Read the model definition and answer for the solid it produces. Units are mm, in the model's axes. A direction names the side the tool comes from. Coordinates: 2 decimals unless noted, no trailing zeros. Loops run counter-clockwise (first coordinate to the right, second up) from the corner with the lowest first, then second, coordinate; pieces in that order, holes last. Notation, with made-up numbers: (47.25, -18.5) - (76.25, -18.5) arc R6 ccw to (76.25, -9.5) - close; hole circle Ø3 at (33.5, -20.75). An arc over 180 degrees is marked (long way). Use one line per item in the form item = value.
from build123d import *

# Parameters (mm, degrees)
F1_DEPTH    = 3.81
F3_T2_ANGLE = 45.4323000541
F2_W        = 20.7137
F2_H        = 2.54
F4_DEPTH    = 30.226
F8_DEPTH    = 20.7137
F9_W        = 10.5537
F9_H        = 7.0042966513
F10_DEPTH   = 51.8170001
F6_W        = 3.81
F6_H        = 40.64
F11_DEPTH   = 10.16


# Not quite as in the source:
# - a fillet or chamfer that OpenCascade refuses, or shapes differently, is made with other operations: its cross-section is extruded or revolved along the edge and cut away or added


with BuildPart() as f1:
    # F0 (on Top) → F1 (new body)
    with BuildSketch(Plane.XY):
        with BuildLine():
            ThreePointArc((32.3535154368, 26.1046796118), (-0.7575616132, 26.3503201986), (-32.5620487044, 17.1373747646))
            Line((-32.5620487044, 17.1373747646), (32.3535154368, 26.1046796118))
        make_face()
        Polygon((32.3535154368, 26.1046796118), (-32.5620487044, 17.1373747646), (-14.3325939581, -32.94764052), (-14.3325939581, -93.2497044648), (21.0546860419, -93.2497044648), align=None)
    extrude(amount=F1_DEPTH)

    # F3: fillet of radius 5.08 on 1 edges, made by hand

    # F3_s1 → F3_t2 (revolve, cut)
    with BuildSketch(Plane(origin=(35.6245782938, -9.4464852648, 0), x_dir=(0, 0, 1), z_dir=(0.966594728, -0.2563096405, 0))):
        with BuildLine():
            ThreePointArc((3.81, -34.1830353327), (1.0639073716, -32.3751984564), (0, -29.2643464831))
            Line((0, -29.2643464831), (0, -34.1830353327))
            Line((0, -34.1830353327), (3.81, -34.1830353327))
        make_face()
    revolve(axis=Axis((14.9550445097, -87.395415893, 0), (0, 0, 1)), revolution_arc=F3_T2_ANGLE, mode=Mode.SUBTRACT)

    # F2 (on face) → F4 (join)
    with BuildSketch(Plane.XY.offset(3.81)):
        with Locations((-0.8633345632, 20.0644456113)):
            Rectangle(F2_W, F2_H)
        with Locations((-0.8633345632, -23.1155543887)):
            Rectangle(F2_W, F2_H)
    extrude(amount=F4_DEPTH)

    # F7 (on face) → F8 (join)
    with BuildSketch(Plane.YZ.offset(9.4935154368)):
        Polygon((-24.3855543887, 40.8603511751), (-24.3855543887, 34.036), (-21.8455543887, 34.036), (-20.6579078442, 34.036), align=None)
        Polygon((17.6067990667, 34.036), (21.3344456113, 34.036), (21.3344456113, 40.8603511751), align=None)
    extrude(amount=-F8_DEPTH)

    # F9 (on face) → F10 (cut, through all)
    with BuildSketch(Plane.XZ.offset(24.3855543887)):
        with Locations((-0.8633345632, 37.3582028494)):
            Rectangle(F9_W, F9_H)
    extrude(amount=-F10_DEPTH, mode=Mode.SUBTRACT)

    # F6 (on face) → F11 (join)
    with BuildSketch(Plane.XY.offset(3.81)):
        with Locations((7.5885154368, -1.5255543887)):
            Rectangle(F6_W, F6_H)
        with Locations((-9.3151845632, -1.5255543887)):
            Rectangle(F6_W, F6_H)
    extrude(amount=F11_DEPTH)


solid = f1.part
Item 1: For a pull along Y with two mould halves and no side action, classify faces 6 (the flat face through (3, -93.25, 2)), 7 (the flat face through (5.684, -2, 9)), 8 (the flat face through (-6.14, 20, 37)) as +Y half, -Y half, draft (parallel to the pull), parting line (faces both ways), or undercut.
Results below:
face_6 = -Y half
face_7 = undercut
face_8 = draft
Item 2: Which of the six approach directions +Z, -Z, +X, -X, +Y, -Y give full straight-line access (tool end or side, diameter ignored) to faces 1 (the flat face through (-1, 18.794, 22)), 2 (the flat face through (-1, -23, 33.856)), 3 (the flat face through (9.494, -3, 13)), 4 (the flat face through (-1, -24.386, 23)), 5 (the flat face through (-14.333, -63, 2))?
Results below:
face_1 = none
face_2 = +Z, +Y, -Y
face_3 = +Z, +X, +Y, -Y
face_4 = +Z, +X, -X, -Y
face_5 = +Z, -Z, -X, -Y
Item 3: Each of these flat-tipped pins is pushed along its axis until it touches: P1, Ø10, axis at x = -18.5, y = -74.5, coming from the +Z side; P2, Ø2, axis at x = -1.5, y = -23.5, coming from the +Z side; P3, Ø1.9, axis at y = -54.5, z = 1.5, coming from the -X side. Where does it stop, or does it pass through?
Results below:
P1 = 3.81
P2 = 33.86
P3 = -14.33
Item 4: The part is cut by section C-C on y = 0. Give the vertices of the cut face in (x, z), plus the area to 3 significant figures.
Results below:
outline = (-26.32, 0) - (29.88, 0) - (29.88, 3.81) - (9.49, 3.81) - (9.49, 13.97) - (5.68, 13.97) - (5.68, 3.81) - (-7.41, 3.81) - (-7.41, 13.97) - (-11.22, 13.97) - (-11.22, 3.81) - (-26.32, 3.81) - close
area = 292 mm²
Item 5: The part is cut by section A-A on z = 29. Give the vertices of the cut face in (x, y), plus the area to 3 significant figures.
Results below:
outline = (-11.22, -24.39) - (9.49, -24.39) - (9.49, -21.85) - (-11.22, -21.85) - close; (-11.22, 18.79) - (9.49, 18.79) - (9.49, 21.33) - (-11.22, 21.33) - close
area = 105 mm²
Item 6: The part is cut by section D-D on y = -56. Give the vertices of the cut face in (x, z).
Results below:
outline = (-14.33, 0) - (24.58, 0) - (24.58, 3.81) - (-14.33, 3.81) - close
Item 7: The part is cut by section B-B on z = 12. Give the vertices of the cut face in (x, y), plus the area to 3 significant figures.
Results below:
outline = (-11.22, -24.39) - (9.49, -24.39) - (9.49, 21.33) - (-11.22, 21.33) - close; hole (-7.41, -21.85) - (5.68, -21.85) - (5.68, 18.79) - (-7.41, 18.79) - close
area = 415 mm²
Item 8: Find the intervals of material crossed by L1, parallel to Y at x = 5, z = 21; L2, parallel to Z at x = 2.5, y = -28; L3, parallel to Y at x = 6, z = 10, in increasing order.
Results below:
L1 = -24.39 to -21.85, 18.79 to 21.33
L2 = 0 to 3.81
L3 = -24.39 to 21.33
